from build123d import *

# Parameters (mm, degrees)
F0_W     = 50
F0_H     = 50
F0_W_2   = 46.8
F0_H_2   = 46.8
F1_DEPTH = 432
F2_W     = 50
F2_H     = 50
F2_W_2   = 46.8
F2_H_2   = 46.8
F3_DEPTH = 75
F4_W     = 50
F4_H     = 50
F4_W_2   = 46.8
F4_H_2   = 46.8
F5_DEPTH = 780


with BuildPart() as f1:
    # F0 (on Top) → F1 (new body)
    with BuildSketch(Plane.XY):
        with Locations((-0.5586, -2.413411)):
            Rectangle(F0_W, F0_H)
        with Locations((-0.5586, -2.413411)):
            Rectangle(F0_W_2, F0_H_2, mode=Mode.SUBTRACT)
    extrude(amount=F1_DEPTH)

    # F2 (on face) → F3 (join)
    with BuildSketch(Plane.YZ.offset(24.4414)):
        with Locations((-2.413411, 50)):
            Rectangle(F2_W, F2_H)
        with Locations((-2.413411, 50)):
            Rectangle(F2_W_2, F2_H_2, mode=Mode.SUBTRACT)
        with Locations((-2.413411, 407)):
            Rectangle(F2_W, F2_H)
        with Locations((-2.413411, 407)):
            Rectangle(F2_W_2, F2_H_2, mode=Mode.SUBTRACT)
    extrude(amount=F3_DEPTH)

    # F4 (on face) → F5 (join)
    with BuildSketch(Plane.XZ.offset(27.413411)):
        with Locations((-0.5586, 407)):
            Rectangle(F4_W, F4_H)
        with Locations((-0.5586, 407)):
            Rectangle(F4_W_2, F4_H_2, mode=Mode.SUBTRACT)
        Polygon((99.4414, 75), (74.4414, 75), (74.4414, 25), (99.4414, 25), (99.4414, 26.6), (76.0414, 26.6), (76.0414, 73.4), (99.4414, 73.4), align=None)
    extrude(amount=F5_DEPTH)

    # F6: F1 across face


with BuildPart() as f1_1:
    add(f1.part)
    add(f1.part.mirror(Plane(origin=(-0.5586, -807.413411, 407), x_dir=(1, 0, 0), z_dir=(0, -1, 0))))

    # F7: F1 across face


with BuildPart() as f1_2:
    add(f1_1.part)
    add(f1_1.part.mirror(Plane(origin=(99.4414, -2.413411, 407), x_dir=(0, 1, 0), z_dir=(1, 0, 0))))


solid = f1_2.part
The listing builds one solid part. Answer for the finished solid, in the listing's coordinates (mm). A direction names the side the tool comes from. Coordinates: 2 decimals unless noted, no trailing zeros. Loops run counter-clockwise (first coordinate to the right, second up) from the corner with the lowest first, then second, coordinate; pieces in that order, holes last. Notation, with made-up numbers: (17, -34.5) -> (71, -34.5) arc R12 ccw to (71, -20.5) -> close; hole circle Ø5 at (68.25, 81.25). An arc over 180 degrees is marked (long way). Write item = value, one per line. Start each with the question number.
1) Given pin 1 Ø4 at (y, z) = (-834.5, 68) entering from -X; pin 2 Ø2 at (x, y) = (117.5, -892) entering from -Z; pin 3 Ø3 at (x, y) = (18, -716) entering from -Z, each flat-ended and moving along its own axis, determine where each tip first touches the part or whether it passes through.
2) The mould has two halves that part along Y. Classify faces 1 (the face through (24.441, -3, 226)), 2 (the face through (174.441, -818, 407)): released by +Y, released by -Y, zero draft, split by the parting line, or undercut.
3) A cutting plane is placed at B-B (y = -607.5). Give the vertices of the cut face in (x, z), then the cut area to 3 significant figures.
4) A cutting plane is placed at C-C (x = 4.5). Give the vertices of the cut face in (y, z), then the cut area to 3 significant figures.
5) A tool of negligible diameter and unlimited length cuts with its end or side. For faces 3 (the face through (200, -1635.813, 213)), 4 (the face through (-3, -26, 0)), 5 (the face through (100, -1612, 430.4)), 6 (the face through (174.441, -3, 226)), from which of +Z, -Z, +X, -X, +Y, -Y can it reach the whole face along a straight path? Write none if from no direction.
6) A cutting plane is placed at A-A (z = 260). Count the separate pieces of the cut face and the enclosed holes in it, then the cut area to 3 significant figures.
7) Straight lines are drawn through the part: line 1 (Y direction, x = 209, z = 146); line 2 (X direction, y = -48, z = 406); line 3 (Z direction, x = -14, y = -428). For each, find the intervals that lie inside material, in ascending order. Write a range as from..to.
Responses:
q1.pin_1 = 74.44
q1.pin_2 = 25
q1.pin_3 = 382
q2.face_1 = zero draft
q2.face_2 = undercut
q3.outline = (-25.56, 382) -> (24.44, 382) -> (24.44, 432) -> (-25.56, 432) -> close; (74.44, 25) -> (124.44, 25) -> (124.44, 75) -> (74.44, 75) -> close; (174.44, 382) -> (224.44, 382) -> (224.44, 432) -> (174.44, 432) -> close; hole (-23.96, 383.6) -> (22.84, 383.6) -> (22.84, 430.4) -> (-23.96, 430.4) -> close; hole (76.04, 26.6) -> (122.84, 26.6) -> (122.84, 73.4) -> (76.04, 73.4) -> close; hole (176.04, 383.6) -> (222.84, 383.6) -> (222.84, 430.4) -> (176.04, 430.4) -> close
q3.area = 929 mm²
q4.outline = (-1637.41, 0) -> (-1635.81, 0) -> (-1635.81, 432) -> (-1637.41, 432) -> close; (-1589.01, 0) -> (-1587.41, 0) -> (-1587.41, 382) -> (-27.41, 382) -> (-27.41, 0) -> (-25.81, 0) -> (-25.81, 432) -> (-1589.01, 432) -> close; (20.99, 0) -> (22.59, 0) -> (22.59, 432) -> (20.99, 432) -> close; hole (-1587.41, 383.6) -> (-27.41, 383.6) -> (-27.41, 430.4) -> (-1587.41, 430.4) -> close
q4.area = 7,760 mm²
q5.face_3 = +Z, -Z
q5.face_4 = -Z, +X, -X, +Y, -Y
q5.face_5 = none
q5.face_6 = +Y, -Y
q6.separate_pieces = 4
q6.enclosed_holes = 4
q6.area = 1,240 mm²
q7.line_1 = -1637.41..-1635.81, -1589.01..-1587.41, -27.41..-25.81, 20.99..22.59
q7.line_2 = -25.56..-23.96, 22.84..24.44, 174.44..176.04, 222.84..224.44
q7.line_3 = 382..383.6, 430.4..432
